from build123d import *

# Parameters (mm, degrees)
F0_R     = 3.9
F1_DEPTH = 16
F2_R     = 2.4
F3_DEPTH = 12
F4_R     = 1.25
F5_DEPTH = 4.001
F6_SIZE  = 0.5
F7_SIZE  = 0.5
F9_DEPTH = 1.6


with BuildPart() as f1:
    # F0 (on Top) → F1 (new body)
    with BuildSketch(Plane.XY):
        Circle(F0_R)
    extrude(amount=F1_DEPTH)

    # F2 (on face) → F3 (cut)
    with BuildSketch(Plane(origin=(0, 0, 0), x_dir=(1, 0, 0), z_dir=(0, 0, -1))):
        Circle(F2_R)
    extrude(amount=-F3_DEPTH, mode=Mode.SUBTRACT)

    # F4 (on face) → F5 (cut, through all)
    with BuildSketch(Plane(origin=(0, 0, 12), x_dir=(1, 0, 0), z_dir=(0, 0, -1))):
        Circle(F4_R)
    extrude(amount=-F5_DEPTH, mode=Mode.SUBTRACT)

    # F6
    f6_edges = [f1.edges().sort_by_distance(p)[0] for p in [
        (-3.9, 0, 16),
    ]]
    chamfer(f6_edges, length=F6_SIZE)

    # F7
    f7_edges = [f1.edges().sort_by_distance(p)[0] for p in [
        (-3.9, 0, 0),
    ]]
    chamfer(f7_edges, length=F7_SIZE)

    # F8 (on face) → F9 (cut)
    with BuildSketch(Plane.XY.offset(16)):
        Polygon((-2.886751, 0), (-1.443376, -2.5), (1.443376, -2.5), (2.886751, 0), (1.443376, 2.5), (-1.443376, 2.5), align=None)
    extrude(amount=-F9_DEPTH, mode=Mode.SUBTRACT)


solid = f1.part
For this review, take the finished solid that the model builds, in its own axes (mm). A direction names the side the tool comes from. Round coordinates to 2 decimals unless told otherwise and drop trailing zeros. Order: outer loops, then holes, each group sorted by start corner. A loop starts at its lowest first (then second) coordinate and runs counter-clockwise, first axis right, second up. Notation, with made-up numbers: M 37,-3 L 57,-3 A21 cw 57,5 Z; hole C 22,50.5 d10. An arc over 180 degrees is marked long. Write each question's results on one line, items separated by ' | '. Start each with the question number.
1. Tool access review of faces 1 (the face through (0, -3, 16)), 2 (the face through (2.175, 1.233, 15.211)), 3 (the face through (1, 1, 12)): name each direction out of +Z, -Z, +X, -X, +Y, -Y from which nothing blocks a thin tool from reaching the whole face with its end or side.
2. To check wall thickness, follow L1, parallel to Y at x = 0, z = 13.55; L2, parallel to Y at x = 0, z = 4; L3, parallel to X at y = -0.5, z = 10.5. State the ranges of each line that lie inside material, in increasing order. Write a range as [from, to].
3. Add section B-B (z = 3.75). State the section outline as (x, y) points.
4. Add section A-A (x = 0). State the section outline as (y, z) points, then the cut area to 3 significant figures.
5. Draft analysis for pull direction Y (two halves, no side actions). For faces 4 (the face through (0, -2.5, 15)), 5 (the face through (-2.87, 2.64, 7.9)), 6 (the face through (1.5, -2.2, 0)), state which applies: pulls with the +Y half, pulls with the -Y half, needs draft (parallel to the pull), parting line crosses it, or undercut.
6. Clearance check with flat-ended pins moving along their axes: pin 1 Ø3 at (x, y) = (0, 0) entering from -Z; pin 2 Ø2 at (x, y) = (0, 0) entering from +Z; pin 3 Ø2 at (y, z) = (3, 6) entering from -X; pin 4 Ø0.5 at (x, z) = (0.5, 15) entering from +Y. State where each tip first meets the part, or that it passes through.
Output values:
1) face 1: +Z, +X, -X, +Y, -Y | face 2: +Z | face 3: -Z
2) L1: [-3.9, -1.25], [1.25, 3.9] | L2: [-3.9, -2.4], [2.4, 3.9] | L3: [-3.87, -2.35], [2.35, 3.87]
3) outline: C 0,0 d7.8; hole C 0,0 d4.8
4) outline: M -3.9,0.5 L -3.4,0 L -2.4,0 L -2.4,12 L -1.25,12 L -1.25,14.4 L -2.5,14.4 L -2.5,16 L -3.4,16 L -3.9,15.5 Z; M 1.25,12 L 2.4,12 L 2.4,0 L 3.4,0 L 3.9,0.5 L 3.9,15.5 L 3.4,16 L 2.5,16 L 2.5,14.4 L 1.25,14.4 Z | area: 52.7 mm^2
5) face 4: undercut | face 5: parting line crosses it | face 6: needs draft
6) pin 1: z = 12 | pin 2: through | pin 3: x = -3.35 | pin 4: y = 3.89
